Read the model definition and answer for the solid it produces. Units are mm, in the model's axes. Round coordinates to 2 decimals unless told otherwise and drop trailing zeros. Write each loop counter-clockwise with the first axis right and the second up, starting at its lowest first coordinate (ties: lowest second). Pieces come first, ordered by that corner, then holes. Notation, with made-up numbers: (8.25, 0.5) - (47.25, 0.5) arc R33 ccw to (47.25, 28.5) - close; hole circle Ø7 at (69.5, 12.5). An arc over 180 degrees is marked (long way). One line per item, written item: value. Start each with the question number.
(1) Find the intervals of material crossed by L1, parallel to Y at x = 30, z = 3.5; L2, parallel to Y at x = 51, z = 6; L3, parallel to Y at x = 14, z = 4, in increasing order.
(2) A cutting plane is placed at D-D, the plane x = 14.5. Determine the outline of the cut face in (y, z), plus the area to 3 significant figures.
(3) A flat-ended cylindrical pin translates along its axis: pin 1 Ø2 at (y, z) = (6, 2.5) entering from +X. Find the tip coordinate at first contact, or state that the pin passes through.
(4) A cutting plane is placed at C-C, the plane y = 29.5. Determine the outline of the cut face in (x, z), plus the area to 4 significant figures.
(5) A cutting plane is placed at B-B, the plane y = 60.5. Determine the outline of the cut face in (x, z).
(6) A cutting plane is placed at A-A, the plane x = 6. Determine the outline of the cut face in (y, z), plus the area to 3 significant figures.
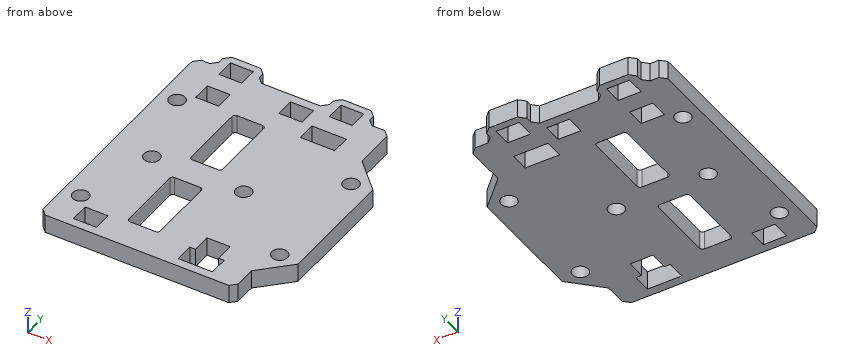
Autodesk Inventor part; units mm, degrees
ref_plane "YZ Plane" through (0, 0, 0) normal (1, 0, 0) x (0, 1, 0)
ref_plane "XZ Plane" through (0, 0, 0) normal (0, 1, 0) x (-1, 0, 0)
ref_plane "XY Plane" through (0, 0, 0) normal (0, 0, 1) x (1, 0, 0)
sketch "Sketch1" plane through (0, 0, 0) normal (0, 0, 1) x (1, 0, 0)
  line L0 (0, 0) -> (68, 0)
  line L1 (68, 87.5) -> (0, 87.5)
  line L2 (0, 87.5) -> (0, 0)
  line L3 (68, 71.5) -> (78, 61.5)
  line L4 (78, 61.5) -> (78, 19.5)
  line L5 (78, 19.5) -> (68, 9.5)
  line L6 (68, 0) -> (68, 9.5)
  line L7 (68, 71.5) -> (68, 87.5)
  line L8 (35, 84.5) -> (43, 84.5)
  line L9 (43, 84.5) -> (43, 78)
  line L10 (43, 78) -> (35, 78)
  line L11 (35, 78) -> (35, 84.5)
  line L12 (10, 78) -> (18, 78)
  line L13 (18, 78) -> (18, 71.5)
  line L14 (18, 71.5) -> (10, 71.5)
  line L15 (10, 71.5) -> (10, 78)
  line L16 (10, 9.5) -> (18, 9.5)
  line L17 (18, 9.5) -> (18, 3)
  line L18 (18, 3) -> (10, 3)
  line L19 (10, 3) -> (10, 9.5)
  line L20 (25, 70.5) -> (34, 70.5)
  line L21 (35, 69.5) -> (35, 46.5)
  line L22 (34, 45.5) -> (25, 45.5)
  line L23 (24, 46.5) -> (24, 69.5)
  line L24 (25, 35.5) -> (34, 35.5)
  line L25 (35, 34.5) -> (35, 11.5)
  line L26 (34, 10.5) -> (25, 10.5)
  line L27 (24, 11.5) -> (24, 34.5)
  arc A0 (25, 70.5) -> (24, 69.5) centre (25, 69.5) ccw
  arc A1 (35, 69.5) -> (34, 70.5) centre (34, 69.5) ccw
  arc A2 (34, 45.5) -> (35, 46.5) centre (34, 46.5) ccw
  arc A3 (24, 46.5) -> (25, 45.5) centre (25, 46.5) ccw
  arc A4 (25, 35.5) -> (24, 34.5) centre (25, 34.5) ccw
  arc A5 (24, 11.5) -> (25, 10.5) centre (25, 11.5) ccw
  arc A6 (34, 10.5) -> (35, 11.5) centre (34, 11.5) ccw
  arc A7 (35, 34.5) -> (34, 35.5) centre (34, 34.5) ccw
  line L28 (29.5, 70.5) -> (29.5, 10.5) construction
  circle A8 centre (71, 60.5) radius 2.75
  circle A9 centre (71, 20.5) radius 2.75
  line L29 (46.5, 3) -> (58.5, 3)
  line L30 (58.5, 3) -> (58.5, 9.5)
  line L31 (58.5, 9.5) -> (46.5, 9.5)
  line L32 (46.5, 9.5) -> (46.5, 3)
  circle A10 centre (6, 13.5) radius 5 construction
  circle A11 centre (6, 13.5) radius 2.75
  circle A12 centre (6, 67.5) radius 5 construction
  circle A13 centre (6, 67.5) radius 2.75
  line L33 (46.5, 78) -> (58.5, 78)
  line L34 (58.5, 78) -> (58.5, 71.5)
  line L35 (58.5, 71.5) -> (46.5, 71.5)
  line L36 (46.5, 71.5) -> (46.5, 78)
  line L37 (21, 84.5) -> (29, 84.5)
  line L38 (29, 84.5) -> (29, 78)
  line L39 (29, 78) -> (21, 78)
  line L40 (21, 78) -> (21, 84.5)
  circle A14 centre (71, 60.5) radius 5 construction
  circle A15 centre (71, 20.5) radius 5 construction
  circle A16 centre (14, 40.5) radius 5 construction
  circle A17 centre (46, 40.5) radius 5 construction
  circle A18 centre (46, 40.5) radius 2.75
  circle A19 centre (14, 40.5) radius 2.75
  line L41 (50, 87.5) -> (50, 0) construction
  line L42 (55, 87.5) -> (55, 0) construction
  line L43 (52.5, 87.5) -> (52.5, 0) construction
  line L44 (72, 13.5) -> (0, 13.5) construction
  line L45 (72, 67.5) -> (0, 67.5) construction
  point P0 (78, 40.5)
  point P1 (52.5, 3)
  dimension "d1" = 45
  dimension "d2" = 10
  dimension "d3" = 6.5
  dimension "d4" = 6.5
  dimension "d5" = 8
  dimension "d6" = 8
  dimension "d7" = 3
  dimension "d8" = 6.5
  dimension "d9" = 3
  dimension "d12" = 1
  dimension "d13" = 11
  dimension "d14" = 25
  dimension "d15" = 25
  dimension "d16" = 1
  dimension "d17" = 1
  dimension "d18" = 38.5
  dimension "d19" = 5.5
  dimension "d20" = 5.5
  dimension "d21" = 7
  dimension "d24" = 12
  dimension "d25" = 11
  dimension "d26" = 11
  dimension "d27" = 10
  dimension "d28" = 5.5
  dimension "d29" = 5.5
  dimension "d30" = 10
  dimension "d32" = 4
  dimension "d33" = 4
  dimension "d34" = 4
  dimension "d35" = 6
  dimension "d36" = 68
  dimension "d39" = 8
  dimension "d40" = 3
  dimension "d41" = 10
  dimension "d42" = 10
  dimension "d43" = 4
  dimension "d44" = 10
  dimension "d45" = 5.5
  dimension "d46" = 10
  dimension "d47" = 5.5
  dimension "d49" = 14
  dimension "d50" = 32
  dimension "d51" = 5
  dimension "d52" = 2.5
  dimension "d53" = 15.5
  dimension "d92" = 4
  dimension "d93" = 4
  dimension "d94" = 54
  dimension "d95" = 6
extrude "Extrusion1" add sketch "Sketch1" along normal blind 6.5
chamfer "Chamfer1" distance 2 angle 45 4 edges at (0, 0, 3.25) (68, 0, 3.25) (68, 87.5, 3.25) (0, 87.5, 3.25)
sketch "Sketch2" plane through (0, 0, 6.5) normal (0, 0, 1) x (1, 0, 0)
  line L0 (46.5, 9.5) -> (58.5, 9.5)
  line L1 (68, 2) -> (68, 9.5)
  line L2 (48.5, 16) -> (56.5, 16)
  line L3 (56.5, 16) -> (56.5, 9.5)
  line L4 (56.5, 9.5) -> (48.5, 9.5)
  line L5 (48.5, 9.5) -> (48.5, 16)
  point P0 (0, 0)
  dimension "d59" = 6.5
  dimension "d60" = 8
  dimension "d63" = 11.5
extrude "Extrusion2" cut sketch "Sketch2" against normal through all
sketch "Sketch3" plane through (0, 0, 6.5) normal (0, 0, 1) x (1, 0, 0)
  line L0 (29, 84.5) -> (29, 78)
  line L1 (29, 78) -> (21, 78)
  line L2 (21, 78) -> (21, 84.5)
  line L3 (21, 84.5) -> (29, 84.5)
  point P0 (0, 0)
extrude "Extrusion3" add sketch "Sketch3" against normal blind 6.5
sketch "Sketch6" plane through (0, 0, 6.5) normal (0, 0, 1) x (1, 0, 0)
  line L0 (18, 78) -> (18, 71.5)
  line L1 (10, 71.5) -> (10, 78)
  line L2 (66, 87.5) -> (2, 87.5)
  line L3 (7, 87.5) -> (21, 87.5)
  line L4 (21, 87.5) -> (21, 93.5)
  line L5 (21, 93.5) -> (7, 93.5)
  line L6 (7, 93.5) -> (7, 87.5)
  line L7 (45.5, 87.5) -> (59.5, 87.5)
  line L8 (59.5, 87.5) -> (59.5, 93.5)
  line L9 (59.5, 93.5) -> (45.5, 93.5)
  line L10 (45.5, 93.5) -> (45.5, 87.5)
  line L11 (46.5, 78) -> (58.5, 78)
  point P0 (0, 0)
  point P1 (52.5, 93.5)
  point P2 (52.5, 78)
  dimension "d80" = 3
  dimension "d81" = 3
  dimension "d84" = 6
extrude "Extrusion6" add sketch "Sketch6" against normal blind 6.5
sketch "Sketch7" plane through (0, 0, 6.5) normal (0, 0, 1) x (1, 0, 0)
  line L0 (18, 78) -> (18, 71.5)
  line L1 (10, 71.5) -> (10, 78)
  line L2 (43, 84.5) -> (43, 78)
  line L3 (35, 78) -> (35, 84.5)
  line L4 (35, 84.5) -> (43, 84.5)
  line L5 (10, 91) -> (18, 91)
  line L6 (18, 91) -> (18, 84.5)
  line L7 (18, 84.5) -> (10, 84.5)
  line L8 (10, 84.5) -> (10, 91)
  line L9 (48.5, 91) -> (56.5, 91)
  line L10 (56.5, 91) -> (56.5, 84.5)
  line L11 (56.5, 84.5) -> (48.5, 84.5)
  line L12 (48.5, 84.5) -> (48.5, 91)
  line L13 (59.5, 93.5) -> (45.5, 93.5)
  point P0 (0, 0)
  point P1 (52.5, 91)
  point P2 (52.5, 93.5)
extrude "Extrusion7" cut sketch "Sketch7" against normal blind 6.5
chamfer "Chamfer3" distance 2 angle 45 8 edges at (7, 87.5, 3.25) (7, 93.5, 3.25) (21, 93.5, 3.25) (21, 87.5, 3.25) (45.5, 87.5, 3.25) (45.5, 93.5, 3.25) (59.5, 93.5, 3.25) (59.5, 87.5, 3.25)
properties part number "x_motor_top" material "Plywood, Finish"
Here are the results:
1. L1: 0 to 10.5, 35.5 to 45.5, 70.5 to 87.5
1. L2: 0 to 3, 16 to 71.5, 78 to 84.5, 91 to 93.5
1. L3: 0 to 3, 9.5 to 37.75, 43.25 to 71.5, 78 to 84.5, 91 to 93.5
2. outline: (0, 0) - (3, 0) - (3, 6.5) - (0, 6.5) - close; (9.5, 0) - (37.8, 0) - (37.8, 6.5) - (9.5, 6.5) - close; (43.2, 0) - (71.5, 0) - (71.5, 6.5) - (43.2, 6.5) - close; (78, 0) - (84.5, 0) - (84.5, 6.5) - (78, 6.5) - close; (91, 0) - (93.5, 0) - (93.5, 6.5) - (91, 6.5) - close
2. area: 446 mm²
3. pin 1: x = 68
4. outline: (0, 0) - (24, 0) - (24, 6.5) - (0, 6.5) - close; (35, 0) - (78, 0) - (78, 6.5) - (35, 6.5) - close
4. area: 435.5 mm²
5. outline: (0, 0) - (24, 0) - (24, 6.5) - (0, 6.5) - close; (35, 0) - (68.25, 0) - (68.25, 6.5) - (35, 6.5) - close; (73.75, 0) - (78, 0) - (78, 6.5) - (73.75, 6.5) - close
6. outline: (0, 0) - (10.75, 0) - (10.75, 6.5) - (0, 6.5) - close; (16.25, 0) - (64.75, 0) - (64.75, 6.5) - (16.25, 6.5) - close; (70.25, 0) - (88.5, 0) - (88.5, 6.5) - (70.25, 6.5) - close
6. area: 504 mm²
